from build123d import *

# Parameters (mm, degrees)
SKETCH_1_W                 = 45
SKETCH_1_H                 = 100
SKETCH_1_W_2               = 3
SKETCH_1_H_2               = 15
EXTRUDE_1_DEPTH            = 1.5
SKETCH_2_W                 = 5.35
SKETCH_2_H                 = 3.2
SKETCH_2_W_2               = 3.3
SKETCH_2_H_2               = 1.4
SKETCH_2_W_3               = 4.35
CUT_EXTRUDE_1_DEPTH        = 57.207205944
MIRROR_2_COPY_1_SKETCH_W   = 5.35
MIRROR_2_COPY_1_SKETCH_H   = 3.2
MIRROR_2_COPY_1_SKETCH_W_2 = 3.3
MIRROR_2_COPY_1_SKETCH_H_2 = 1.4
MIRROR_2_COPY_1_SKETCH_W_3 = 4.35
MIRROR_2_COPY_1_DEPTH      = 57.207205944


with BuildPart() as part:
    # 草图1 → 凸台-拉伸1 (new, symmetric)
    with BuildSketch(Plane(origin=(0, 0, 0), x_dir=(1, 0, 0), z_dir=(0, 1, 0))):
        Rectangle(SKETCH_1_W, SKETCH_1_H)
        with Locations((-24, 25)):
            Rectangle(SKETCH_1_W_2, SKETCH_1_H_2)
        with Locations((-24, -25)):
            Rectangle(SKETCH_1_W_2, SKETCH_1_H_2)
        with Locations((24, -25)):
            Rectangle(SKETCH_1_W_2, SKETCH_1_H_2)
        with Locations((24, 25)):
            Rectangle(SKETCH_1_W_2, SKETCH_1_H_2)
    extrude(amount=EXTRUDE_1_DEPTH, both=True)

    # 草图2 → 切除-拉伸1 (cut, symmetric)
    with BuildSketch(Plane(origin=(0, 1.5, 0), x_dir=(1, 0, 0), z_dir=(0, 1, 0))):
        with Locations((15.175, 25)):
            Rectangle(SKETCH_2_W, SKETCH_2_H)
        with Locations((19.5, 27.3)):
            Rectangle(SKETCH_2_W_2, SKETCH_2_H_2)
        with Locations((19.5, 25)):
            Rectangle(SKETCH_2_W_2, SKETCH_2_H)
        with Locations((19.5, 22.7)):
            Rectangle(SKETCH_2_W_2, SKETCH_2_H_2)
        with Locations((23.325, 25)):
            Rectangle(SKETCH_2_W_3, SKETCH_2_H)
    cut_extrude_1 = extrude(amount=CUT_EXTRUDE_1_DEPTH, both=True, mode=Mode.SUBTRACT)

    # 镜向1: 切除-拉伸1 across plane
    add(cut_extrude_1.mirror(Plane(origin=(0, 0, 0), x_dir=(0, 0, 1), z_dir=(1, 0, 0))), mode=Mode.SUBTRACT)

    # 镜向2: 切除-拉伸1 across plane
    add(cut_extrude_1.mirror(Plane.XY), mode=Mode.SUBTRACT)

    # 镜向2 copy 1 sketch → 镜向2 copy 1 (cut, symmetric)
    with BuildSketch(Plane(origin=(0, 1.5, 0), x_dir=(-1, 0, 0), z_dir=(0, 1, 0))):
        with Locations((15.175, 25)):
            Rectangle(MIRROR_2_COPY_1_SKETCH_W, MIRROR_2_COPY_1_SKETCH_H)
        with Locations((19.5, 27.3)):
            Rectangle(MIRROR_2_COPY_1_SKETCH_W_2, MIRROR_2_COPY_1_SKETCH_H_2)
        with Locations((19.5, 25)):
            Rectangle(MIRROR_2_COPY_1_SKETCH_W_2, MIRROR_2_COPY_1_SKETCH_H)
        with Locations((19.5, 22.7)):
            Rectangle(MIRROR_2_COPY_1_SKETCH_W_2, MIRROR_2_COPY_1_SKETCH_H_2)
        with Locations((23.325, 25)):
            Rectangle(MIRROR_2_COPY_1_SKETCH_W_3, MIRROR_2_COPY_1_SKETCH_H)
    extrude(amount=MIRROR_2_COPY_1_DEPTH, both=True, mode=Mode.SUBTRACT)


solid = part.part
For this review, take the finished solid that the model builds, in its own axes (mm). A direction names the side the tool comes from. Give positions to 0.01 mm unless a question says otherwise; leave off trailing zeros. Loops run counter-clockwise (first coordinate to the right, second up) from the corner with the lowest first, then second, coordinate; pieces in that order, holes last.
Item 1: Take a section at B-B, the plane x = -16.5. State the section outline as (y, z) points, and give its area (3 significant figures).
Item 2: Draft analysis for pull direction Z (two halves, no side actions). For faces 1 (the flat face through (-25.5, 0, 30)), 2 (the flat face through (-24, 0, 32.5)), 3 (the flat face through (-19, 0, 28)), 4 (the flat face through (-19, 0, -22)), state which applies: +Z half, -Z half, draft (parallel to the pull), parting line (faces both ways), or undercut.
Item 3: Take a section at A-A, the plane x = 20. State the section outline as (y, z) points, and give its area (3 significant figures).
Item 4: Insertion check: pin 1 (0.9 mm diameter, centred on x = 24, y = 0.5, fed in from -Z); pin 2 (1.5 mm diameter, centred on y = 0.5, z = 41, fed in from +X); pin 3 (0.9 mm diameter, centred on y = -0.5, z = 37, fed in from -X). Each pin has a flat end and moves straight along its axis. Give the tip position at first contact, or say it passes through.
Item 5: Take a section at C-C, the plane z = 42. State the section outline as (x, y) points, and give its area (3 significant figures).
Item 6: Tool access review of faces 5 (the flat face through (22.5, 0, 0)), 6 (the flat face through (-24, 0, -17.5)), 7 (the flat face through (-25.5, 0, 20)), 8 (the flat face through (0, 0, -50)), 9 (the flat face through (-19, 0, 22)): name each direction out of +Z, -Z, +X, -X, +Y, -Y from which nothing blocks a thin tool from reaching the whole face with its end or side.
Item 7: For line 1 along Z through (x, y) = (17.5, -1.25); line 2 along Z through (x, y) = (-20.5, 1.45); line 3 along X through (y, z) = (0, -22.5), list the stretches that pass through material, from the lowest coordinate up.
Calculated:
1. outline: (-1.5, -50) - (1.5, -50) - (1.5, -26.6) - (-1.5, -26.6) - close; (-1.5, -23.4) - (1.5, -23.4) - (1.5, 23.4) - (-1.5, 23.4) - close; (-1.5, 26.6) - (1.5, 26.6) - (1.5, 50) - (-1.5, 50) - close
1. area: 281 mm2
2. face 1: draft
2. face 2: +Z half
2. face 3: undercut
2. face 4: undercut
3. outline: (-1.5, -50) - (1.5, -50) - (1.5, -28) - (-1.5, -28) - close; (-1.5, -22) - (1.5, -22) - (1.5, 22) - (-1.5, 22) - close; (-1.5, 28) - (1.5, 28) - (1.5, 50) - (-1.5, 50) - close
3. area: 264 mm2
4. pin 1: stops at z = -32.5
4. pin 2: stops at x = 22.5
4. pin 3: stops at x = -22.5
5. outline: (-22.5, -1.5) - (22.5, -1.5) - (22.5, 1.5) - (-22.5, 1.5) - close
5. area: 135 mm2
6. face 5: +X, +Y, -Y
6. face 6: -X, +Y, -Y
6. face 7: +Z, -Z, -X, +Y, -Y
6. face 8: -Z, +X, -X, +Y, -Y
6. face 9: +Y, -Y
7. line 1: z = -50 to -26.6, -23.4 to 23.4, 26.6 to 50
7. line 2: z = -50 to -28, -22 to 22, 28 to 50
7. line 3: x = -25.5 to -21.15, -17.85 to 17.85, 21.15 to 25.5
